The listing builds one solid part. Answer for the finished solid, in the listing's coordinates (mm). A direction names the side the tool comes from. Round coordinates to 2 decimals unless told otherwise and drop trailing zeros. Loops run counter-clockwise (first coordinate to the right, second up) from the corner with the lowest first, then second, coordinate; pieces in that order, holes last. Notation, with made-up numbers: M 87.5,60.5 L 146.5,60.5 A7 ccw 146.5,73.5 Z; hole C -17,-8.75 d1. An arc over 180 degrees is marked long. Answer as a JSON object with one key per item and string values.
```python
from build123d import *

# Parameters (mm, degrees)
CUT_EXTRUDE1_DEPTH = 206.0000001


with BuildPart() as part:
    # Sketch1 → Loft4 section 0
    with BuildSketch(Plane(origin=(0, 0, 0), x_dir=(0, 0, -1), z_dir=(1, 0, 0))):
        Polygon((-205, 400), (195, 400), (195, 390), (0, 390), (0, -390), (195, -390), (195, -400), (-205, -400), (-205, -390), (-10, -390), (-10, 390), (-205, 390), align=None)
    # Sketch4 → Loft4 section 1
    with BuildSketch(Plane(origin=(1000, 0, -1000), x_dir=(0, 0, 1), z_dir=(-1, 0, 0))):
        Polygon((805, 300), (1205, 300), (1205, 290), (1010, 290), (1010, -290), (1205, -290), (1205, -300), (805, -300), (805, -290), (1000, -290), (1000, 290), (805, 290), align=None)
    loft()

    # Sketch6 → Cut-Extrude1 (cut, through all)
    with BuildSketch(Plane.XY.offset(10)):
        with BuildLine():
            Line((221.736940013, 233.917126741), (878.189220239, -166.0970465))
            ThreePointArc((878.189220239, -166.0970465), (908.491436403, -166.635109102), (923.8, -140.478624315))
            Line((923.8, -140.478624315), (923.8, 193.890320904))
            ThreePointArc((923.8, 193.890320904), (916.043576007, 214.020480527), (896.785111571, 223.74143661))
            Line((896.785111571, 223.74143661), (240.332831344, 289.386664633))
            ThreePointArc((240.332831344, 289.386664633), (208.903576567, 269.071308844), (221.736940013, 233.917126741))
        make_face()
        with BuildLine():
            Line((121.727711267, 245.109508509), (819.804188988, -177.17381685))
            ThreePointArc((819.804188988, -177.17381685), (833.539047237, -209.453423865), (807.261589291, -232.693788838))
            Line((807.261589291, -232.693788838), (109.185111571, -302.50143661))
            ThreePointArc((109.185111571, -302.50143661), (86.069840377, -294.89389691), (76.2, -272.650320904))
            Line((76.2, -272.650320904), (76.2, 219.440652228))
            ThreePointArc((76.2, 219.440652228), (91.466218035, 245.573307451), (121.727711267, 245.109508509))
        make_face()
    extrude(amount=-CUT_EXTRUDE1_DEPTH, mode=Mode.SUBTRACT)


solid = part.part
```
Item 1: The part is cut by section A-A (z = -34.5). Give the vertices of the cut face in (x, y), then the cut area to 3 significant figures.
Values follow:
{"outline": "M 0,-400 L 1000,-300 L 1000,-290 L 0,-390 Z; M 0,390 L 1000,290 L 1000,300 L 0,400 Z", "area": "20,000 mm^2"}
Item 2: Flat-ended cylindrical pins translate along their axes: P1, Ø1.5, axis at x = 200.5, z = 131.5, coming from the +Y side (3 decimals); P2, Ø1.5, axis at x = 231.5, z = -143.5, coming from the -Y side (3 decimals); P3, Ø2, axis at x = 627.5, z = 77.5, coming from the +Y side. Find the tip coordinate at first contact, or state that the pin passes through.
Values follow:
{"P1": "y = 380.025", "P2": "y = -376.925", "P3": "y = 337.35"}
Item 3: Which of the six approach directions +Z, -Z, +X, -X, +Y, -Y give full straight-line access (tool end or side, diameter ignored) to faces 4 (the face through (908.1, -166.85, 5.07)), 5 (the face through (0, 115, 1)), 6 (the face through (507, 339.3, -98.9)), 7 (the face through (507, -339.3, 108.9))?
Values follow:
{"face 4": "+Z, -Z", "face 5": "+Z, -Z, -X, +Y, -Y", "face 6": "-Z, -X", "face 7": "+Z, -X"}
Item 4: The part is cut by section B-B (y = 156.5). Give the number of separate pieces and of enclosed holes in the cut face, then the cut area to 3 significant figures.
Values follow:
{"separate pieces": "3", "enclosed holes": "0", "area": "2,330 mm^2"}
Item 5: Straight lines are drawn through the part: line 1 (Z direction, x = 763.5, y = 305); line 2 (Y direction, x = 675.5, z = -129.5); line 3 (Y direction, x = 897, z = -63). For each, find the intervals that lie inside material, in ascending order.
Values follow:
{"line 1": "0 to 10", "line 2": "-332.45 to -322.45, 322.45 to 332.45", "line 3": "-310.3 to -300.3, 300.3 to 310.3"}
Item 6: Determine the mould class of faces 1 (the face through (507, -339.3, -96.1)), 2 (the face through (465.879, 36.924, 5.07)), 3 (the face through (1000, 2, 5)) for opening direction X: released by +X, released by -X, zero draft, split by the parting line, or undercut.
Values follow:
{"face 1": "released by -X", "face 2": "undercut", "face 3": "released by +X"}
